from build123d import *

# Parameters (mm, degrees)
SKETCH1_R                  = 7
SKETCH1_R_2                = 4
BOSS_EXTRUDE1_DEPTH        = 3.5
M4X0_7_TAPPED_HOLE1_REACH  = 18.039
M4X0_7_TAPPED_HOLE1_BORE_R = 1.65
CHAMFER1_SIZE              = 0.5


with BuildPart() as part:
    # Sketch1 → Boss-Extrude1 (new, symmetric)
    with BuildSketch(Plane(origin=(0, 0, 0), x_dir=(1, 0, 0), z_dir=(0, 1, 0))):
        with Locations(Location((0, 0, 0), (0, 0, 270))):
            Circle(SKETCH1_R)
        with Locations(Location((0, 0, 0), (0, 0, 270))):
            Circle(SKETCH1_R_2, mode=Mode.SUBTRACT)
    extrude(amount=BOSS_EXTRUDE1_DEPTH, both=True)

    # M4x0.7 Tapped Hole1 bore → M4x0.7 Tapped Hole1 (cut, up to next)
    with BuildSketch(Plane.XY.offset(7), mode=Mode.PRIVATE) as m4x0_7_tapped_hole1_sk1:
        Circle(M4X0_7_TAPPED_HOLE1_BORE_R)
    m4x0_7_tapped_hole1_tool1 = extrude(m4x0_7_tapped_hole1_sk1.sketch, amount=-M4X0_7_TAPPED_HOLE1_REACH, mode=Mode.PRIVATE) & part.part
    add(m4x0_7_tapped_hole1_tool1.solids().sort_by_distance((0, 0, 7))[0], mode=Mode.SUBTRACT)

    # Chamfer1
    chamfer1_edges = [part.edges().sort_by_distance(p)[0] for p in [
        (0, -3.5, -7),
        (0, 3.5, -7),
    ]]
    chamfer(chamfer1_edges, length=CHAMFER1_SIZE)


solid = part.part
The listing builds one solid part. Answer for the finished solid, in the listing's coordinates (mm). Give positions to 0.01 mm unless a question says otherwise; leave off trailing zeros. Order: outer loops, then holes, each group sorted by start corner. A loop starts at its lowest first (then second) coordinate and runs counter-clockwise, first axis right, second up. Notation, with made-up numbers: (-29, 8) - (27, 8) arc R16 cw to (27, 12) - close; hole circle Ø3 at (60.5, 80). An arc over 180 degrees is marked (long way). Answer as CSV lines item,"result".
Q1. A cutting plane is placed at B-B, the plane z = 0. Determine the outline of the cut face in (x, y), and give its area (3 significant figures).
Answer key:
outline,"(-7, -3) - (-6.5, -3.5) - (-4, -3.5) - (-4, 3.5) - (-6.5, 3.5) - (-7, 3) - close; (4, -3.5) - (6.5, -3.5) - (7, -3) - (7, 3) - (6.5, 3.5) - (4, 3.5) - close"
area,"41.5 mm^2"
Q2. Straight lines are drawn through the part: L1, parallel to Y at x = 0, z = 5.6; L2, parallel to X at y = -1.5, z = 0; L3, parallel to X at y = 0, z = 5.4. For each, find the intervals that lie inside material, in ascending order.
Answer key:
L1,"y = -3.5 to -1.65, 1.65 to 3.5"
L2,"x = -7 to -4, 4 to 7"
L3,"x = -4.45 to -1.65, 1.65 to 4.45"
Q3. A cutting plane is placed at A-A, the plane x = 0. Determine the outline of the cut face in (y, z), and give its area (3 significant figures).
Answer key:
outline,"(-3.5, -6.5) - (-3, -7) - (3, -7) - (3.5, -6.5) - (3.5, -4) - (-3.5, -4) - close; (-3.5, 4) - (-1.65, 4) - (-1.65, 7) - (-3, 7) - (-3.5, 6.5) - close; (1.65, 4) - (3.5, 4) - (3.5, 6.5) - (3, 7) - (1.65, 7) - close"
area,"31.6 mm^2"
Q4. A cutting plane is placed at D-D, the plane y = 1. Determine the outline of the cut face in (x, z), and give its area (3 significant figures).
Answer key:
outline,"(-1.31, 3.78) - (-1.31, 6.88) arc R7 ccw (long way) to (1.31, 6.88) - (1.31, 3.78) arc R4 cw (long way) to start"
area,"95.7 mm^2"
Q5. A cutting plane is placed at C-C, the plane y = -2. Determine the outline of the cut face in (x, z).
Answer key:
outline,"circle Ø14 at (0, 0); hole circle Ø8 at (0, 0)"
Q6. Each of these flat-tipped pins is pushed along its axis until it touches: pin 1 Ø7 at (x, z) = (0, 0) entering from -Y; pin 2 Ø2 at (y, z) = (2, 2) entering from -X. Where does it stop, or does it pass through?
Answer key:
pin 1,"passes through"
pin 2,"stops at x = -6.93"
Q7. Determine the mould class of faces 1 (the face through (3, 3.5, 3)), 2 (the face through (-1.65, 0.07, 5.35)), 3 (the face through (3, -3.5, 3)) for opening direction Y: pulls with the +Y half, pulls with the -Y half, needs draft (parallel to the pull), parting line crosses it, or undercut.
Answer key:
face 1,"pulls with the +Y half"
face 2,"undercut"
face 3,"pulls with the -Y half"
